from build123d import *

# Parameters (mm, degrees)
SKETCH1_W           = 24
SKETCH1_H           = 12
BOSS_EXTRUDE1_DEPTH = 1.5
SKETCH2_W           = 6.5
SKETCH2_H           = 5.5
BOSS_EXTRUDE2_DEPTH = 3
SKETCH6_R           = 1.325
CUT_EXTRUDE1_DEPTH  = 17.552945357
SKETCH7_R           = 1.325
CUT_EXTRUDE2_DEPTH  = 17.552945357
FILLET1_R           = 3.5
FILLET2_R           = 5
FILLET3_R           = 1
FILLET5_R           = 1
SKETCH8_R           = 0.875
CUT_EXTRUDE4_DEPTH  = 16.882380341


# Some blends are built 0.0001 mm under size
with BuildPart() as part:
    # Sketch1 → Boss-Extrude1 (new, symmetric)
    with BuildSketch(Plane.XY):
        Rectangle(SKETCH1_W, SKETCH1_H)
    extrude(amount=BOSS_EXTRUDE1_DEPTH, both=True)

    # Sketch2 → Boss-Extrude2 (add)
    with BuildSketch(Plane(origin=(0, 6, 0), x_dir=(1, 0, 0), z_dir=(0, 1, 0))):
        with Locations((8.75, 4.25)):
            Rectangle(SKETCH2_W, SKETCH2_H)
        with Locations((-8.75, 4.25)):
            Rectangle(SKETCH2_W, SKETCH2_H)
    extrude(amount=-BOSS_EXTRUDE2_DEPTH)

    # Sketch6 → Cut-Extrude1 (cut, through all)
    with BuildSketch(Plane.XZ.offset(-3)):
        with Locations(Location((-8.75, -3.5, 0), (0, 0, 270))):
            Circle(SKETCH6_R)
    extrude(amount=-CUT_EXTRUDE1_DEPTH, mode=Mode.SUBTRACT)

    # Sketch7 → Cut-Extrude2 (cut, through all)
    with BuildSketch(Plane.XZ.offset(-3)):
        with Locations(Location((8.75, -3.5, 0), (0, 0, 270))):
            Circle(SKETCH7_R)
    extrude(amount=-CUT_EXTRUDE2_DEPTH, mode=Mode.SUBTRACT)

    # Fillet1
    # the kernel refuses this fillet: 3.5 mm, written as the material it adds along each edge
    with BuildSketch(Plane(origin=(5.5, 3, -1.5), x_dir=(0, -1, 0), z_dir=(1, 0, 0))) as fillet1_piece_1_section:
        with BuildLine():
            CenterArc((FILLET1_R, FILLET1_R), FILLET1_R, 180, 90)
            Line((0, FILLET1_R), (0, 0))
            Line((0, 0), (FILLET1_R, 0))
        make_face()
    fillet1_piece_1 = extrude(amount=6.5, mode=Mode.PRIVATE)
    fillet1_piece_1 = fillet1_piece_1 - Plane(origin=(8.75, 2.130609202, -3.5), x_dir=(0, 0, -1), z_dir=(0, -1, 0)) * Cylinder(1.325, 27, mode=Mode.PRIVATE)
    add(fillet1_piece_1)
    with BuildSketch(Plane(origin=(-12, 3, -1.5), x_dir=(0, -1, 0), z_dir=(1, 0, 0))) as fillet1_piece_2_section:
        with BuildLine():
            CenterArc((FILLET1_R, FILLET1_R), FILLET1_R, 180, 90)
            Line((0, FILLET1_R), (0, 0))
            Line((0, 0), (FILLET1_R, 0))
        make_face()
    fillet1_piece_2 = extrude(amount=6.5, mode=Mode.PRIVATE)
    fillet1_piece_2 = fillet1_piece_2 - Plane(origin=(-8.75, 2.130609202, -3.5), x_dir=(0, 0, -1), z_dir=(0, -1, 0)) * Cylinder(1.325, 27, mode=Mode.PRIVATE)
    add(fillet1_piece_2)

    # Fillet2
    fillet2_edges = [part.edges().sort_by_distance(p)[0] for p in [
        (5.5, 2.75, -1.5),
        (-5.5, 2.75, -1.5),
    ]]
    fillet(fillet2_edges, radius=FILLET2_R)

    # Fillet3
    fillet3_edges = [part.edges().sort_by_distance(p)[0] for p in [
        (12, 4.5, -7),
        (-12, 4.5, -7),
        (5.5, 4.5, -7),
        (-5.5, 4.5, -7),
    ]]
    fillet(fillet3_edges, radius=FILLET3_R)

    # Fillet5
    fillet5_edges = [part.edges().sort_by_distance(p)[0] for p in [
        (8.739565186, 3, -7),
        (11.707106781, 3, -6.707106781),
        (5.802129531, 3, -6.735982243),
        (-5.406145562, 3, -5.535771954),
        (-8.739565186, 3, -7),
        (-11.707106781, 3, -6.707106781),
        (-5.802129531, 3, -6.735982243),
        (-12, 0, 1.5),
        (12, 0, 1.5),
        (12, 3, -5.5),
        (-12, -3.25, -1.5),
        (-12, 3, -5.5),
        (12, 1.974873734, -2.525126266),
        (-12, 1.974873734, -2.525126266),
        (12, -3.25, -1.5),
        (3.087209053, 1.628244963, -2.221408019),
        (5.406145562, 3, -5.535771954),
        (-3.087209053, 1.628244963, -2.221408019),
    ]]
    fillet(fillet5_edges, radius=FILLET5_R - 0.0004)  # a hair under: the kernel refuses the full size

    # Sketch8 → Cut-Extrude4 (cut, through all)
    with BuildSketch(Plane.XY.offset(1.5)):
        with Locations((7, 1)):
            Circle(SKETCH8_R)
        with Locations((-7, 1)):
            Circle(SKETCH8_R)
    extrude(amount=-CUT_EXTRUDE4_DEPTH, mode=Mode.SUBTRACT)


solid = part.part
Verification items for the finished model (mm, model axes). A direction names the side the tool comes from. Round coordinates to 2 decimals unless told otherwise and drop trailing zeros. Order: outer loops, then holes, each group sorted by start corner. A loop starts at its lowest first (then second) coordinate and runs counter-clockwise, first axis right, second up.
1. Section check D-D on y = 1. State how many separate pieces and enclosed holes the cut face has, then the cut area to 3 significant figures.
Final values:
separate pieces: 3
enclosed holes: 0
area: 66.3 mm2
2. Access from +Z, -Z, +X, -X, +Y, -Y to the whole of each face (thin tool, end or side, straight path). Record for faces 4 (the cylindrical face through (11.715, 3.301, -5.493)), 5 (the cylindrical face through (3.277, 4.24, -2.342)), 6 (the flat face through (-8.7, 3, -5.5)).
Final values:
face 4: -Z, +X, -Y
face 5: -Z, +Y, -Y
face 6: -Z, +X, -X, -Y
3. Release check for a two-part mould opening along Y. For faces 1 (the flat face through (0, 6, -1)), 2 (the cylindrical face through (-7.11, 1.87, -0.01)), 3 (the cylindrical face through (11.715, -3.288, -1.199)) record: +Y half, -Y half, draft (parallel to the pull), parting line (faces both ways), or undercut.
Final values:
face 1: +Y half
face 2: undercut
face 3: draft
4. Go/stop test with flat-tipped pins: P1, Ø1.1, axis at x = -9, z = -5.5, coming from the -Y side; P2, Ø2, axis at x = 7, y = 1, coming from the -Z side. Record where each tip stops, or that it passes through.
Final values:
P1: stops at y = 3
P2: stops at z = -2.55
5. Section check C-C on z = 1. Record the cut outline in (x, y) (3 decimals).
Final values:
outline: (-11.866, -6) - (11.866, -6) - (11.866, 6) - (-11.866, 6) - close; hole circle Ø1.75 at (-7, 1); hole circle Ø1.75 at (7, 1)
6. Section check B-B on y = -4. Record the cut outline in (x, z), then the cut area to 3 significant figures.
Final values:
outline: (-12, -0.5) arc R1 ccw to (-11, -1.5) - (11, -1.5) arc R1 ccw to (12, -0.5) - (12, 0.5) arc R1 ccw to (11, 1.5) - (-11, 1.5) arc R1 ccw to (-12, 0.5) - close
area: 71.1 mm2
7. Thickness scan on L1, parallel to X at y = 3.5, z = -3.25; L2, parallel to Z at x = -8.75, y = 4.45 (3 decimals); L3, parallel to Z at x = -11, y = -1.5. Record the ranges inside material, lowest first.
Final values:
L1: x = -11.99 to -10.05, -7.45 to -4.3, 4.3 to 7.45, 10.05 to 11.99
L2: z = -7 to -4.825, -2.175 to 1.5
L3: z = -1.5 to 1.5
8. Section check A-A on x = -8.75. Record the cut outline in (y, z) (3 decimals).
Final values:
outline: (-6, -1.5) - (-0.5, -1.5) arc R3.5 cw to (1.566, -2.175) - (6, -2.175) - (6, 1.5) - (-6, 1.5) - close; (2.996, -4.825) arc R3.5 cw to (3, -5) - (3, -6) arc R1 ccw to (4, -7) - (6, -7) - (6, -4.825) - close
